Check sheet for the modelled part. Datum: model origin and axes. Units: mm. A direction names the side the tool comes from. Round coordinates to 2 decimals unless told otherwise and drop trailing zeros. Order: outer loops, then holes, each group sorted by start corner. A loop starts at its lowest first (then second) coordinate and runs counter-clockwise, first axis right, second up.
Autodesk Inventor part; units mm, degrees
ref_plane "YZ Plane" through (0, 0, 0) normal (1, 0, 0) x (0, 1, 0)
ref_plane "XZ Plane" through (0, 0, 0) normal (0, 1, 0) x (-1, 0, 0)
ref_plane "XY Plane" through (0, 0, 0) normal (0, 0, 1) x (1, 0, 0)
sketch "Esquisse1" plane through (0, 0, 0) normal (0, 0, 1) x (1, 0, 0)
  circle A0 centre (0, 0) radius 16.5
  dimension "d0" = 33
extrude "Extrusion1" add sketch "Esquisse1" along normal blind 32
sketch "Esquisse2" plane through (0, 0, 32) normal (0, 0, 1) x (1, 0, 0)
  circle A0 centre (0, 0) radius 4
  dimension "d3" = 8
extrude "Extrusion2" cut sketch "Esquisse2" against normal through all
chamfer "Chanfrein1" distance 9 distance2 30 1 edges at (-16.5, 0, 32) measured on face at (12.1348, -1.6353, 32)
sketch "Esquisse3" plane through (0, 0, 32) normal (0, 0, 1) x (1, 0, 0)
  line L0 (2.5, 6) -> (2.5, 16.5)
  line L1 (6, 2.5) -> (16.5, 2.5)
  arc A0 (6, 2.5) -> (2.5, 6) centre (0, 0) ccw
  arc A1 (16.5, 2.5) -> (2.5, 16.5) centre (0, 0) ccw
  dimension "d9" = 2.5
  dimension "d10" = 2.5
  dimension "d11" = 6
  dimension "d12" = 16.5
extrude "Extrusion3" cut sketch "Esquisse3" against normal blind 30
pattern_circular "Réseau circulaire1" count 4 over 360 about axis through (0, 0, 32) along (0, 0, -1) of "Extrusion3"
sketch "Esquisse4" plane through (-16.3095, 2.5, 2) normal (0, 0, 1) x (1, 0, 0)
  circle A0 centre (8.8095, 5) radius 1.6
  point P0 (16.3095, -2.5)
  dimension "d18" = 3.2
  dimension "d19" = 7.5
  dimension "d20" = 7.5
extrude "Extrusion4" cut sketch "Esquisse4" against normal through all
pattern_circular "Réseau circulaire2" count 4 over 360 about axis through (0, 0, 32) along (0, 0, -1) of "Extrusion4"
properties part number "PieddeMat" material "Plastique ABS"
Item 1: Access from +Z, -Z, +X, -X, +Y, -Y to the whole of each face (thin tool, end or side, straight path). Record for faces 4 (the flat face through (9.3, 8, 2)), 5 (the flat face through (-2.5, -10, 14)), 6 (the cylindrical face through (4.57, -4.62, 17.21)), 7 (the flat face through (-8, 9.3, 2)), 8 (the conical face through (-0.053, 11.063, 20.123)).
Answer:
face 4: +Z, +X, +Y
face 5: +Z, -X, -Y
face 6: +Z, +X, -Y
face 7: +Z, -X, +Y
face 8: +Z, +Y
Item 2: Go/stop test with flat-tipped pins: P1, Ø5, axis at x = 9, z = 17.5, coming from the -Y side; P2, Ø11, axis at x = -9, y = 8.5, coming from the +Z side; P3, Ø3, axis at y = -9.5, z = 17, coming from the -X side. Record where each tip stops, or that it passes through.
Answer:
P1: stops at y = -2.5
P2: stops at z = 2
P3: stops at x = -2.5
Item 3: Sectioned sample at B-B (z = 29.5). Record the cut outline in (x, y).
Answer:
outline: (-7.86, -2.5) - (-6, -2.5) arc R6.5 ccw to (-2.5, -6) - (-2.5, -7.86) arc R8.25 ccw to (2.5, -7.86) - (2.5, -6) arc R6.5 ccw to (6, -2.5) - (7.86, -2.5) arc R8.25 ccw to (7.86, 2.5) - (6, 2.5) arc R6.5 ccw to (2.5, 6) - (2.5, 7.86) arc R8.25 ccw to (-2.5, 7.86) - (-2.5, 6) arc R6.5 ccw to (-6, 2.5) - (-7.86, 2.5) arc R8.25 ccw to start; hole circle Ø8 at (0, 0)
Item 4: Scan lines: line 1 along Y through (x, z) = (-7.5, 0.55); line 2 along Y through (x, z) = (6.5, 26); line 3 along Z through (x, y) = (3, 15). Record each from-to range of solid material in increasing order.
Answer:
line 1: y = -14.7 to -9.1, -5.9 to 5.9, 9.1 to 14.7
line 2: y = -2.5 to 2.5
line 3: z = 0 to 2
Item 5: Sectioned sample at A-A (y = 0). Record the cut outline in (x, z).
Answer:
outline: (-16.5, 0) - (-4, 0) - (-4, 32) - (-7.5, 32) - (-16.5, 2) - close; (4, 0) - (16.5, 0) - (16.5, 2) - (7.5, 32) - (4, 32) - close
Item 6: Release check for a two-part mould opening along X. For faces 1 (the cylindrical face through (15.24, 6.32, 0.99)), 2 (the cylindrical face through (-0.867, -3.905, 16.224)), 3 (the flat face through (-10, -2.5, 14)) record: released by +X, released by -X, zero draft, split by the parting line, or undercut.
Answer:
face 1: split by the parting line
face 2: undercut
face 3: zero draft
Item 7: Sectioned sample at C-C (y = -6.5). Record the cut outline in (x, z).
Answer:
outline: (-15.17, 0) - (-8.75, 0) - (-8.75, 2) - (-15.17, 2) - close; (-6.25, 0) - (6.25, 0) - (6.25, 2) - (2.5, 2) - (2.5, 32) - (-2.5, 32) - (-2.5, 2) - (-6.25, 2) - close; (8.75, 0) - (15.17, 0) - (15.17, 2) - (8.75, 2) - close
Item 8: Sectioned sample at D-D (x = 8.5). State how many separate pieces and enclosed holes the cut face has, and give its area (3 significant figures).
Answer:
separate pieces: 3
enclosed holes: 0
area: 178 mm2
